Autodesk Inventor part; units mm, degrees
ref_plane "YZ Plane" through (0, 0, 0) normal (1, 0, 0) x (0, 1, 0)
ref_plane "XZ Plane" through (0, 0, 0) normal (0, 1, 0) x (-1, 0, 0)
ref_plane "XY Plane" through (0, 0, 0) normal (0, 0, 1) x (1, 0, 0)
sketch "Sketch1" plane through (0, 0, 0) normal (1, 0, 0) x (0, 1, 0)
  circle A0 centre (0, 0) radius 44
  dimension "d0" = 88
extrude "Extrusion1" add sketch "Sketch1" along normal blind 3.5
sketch "Sketch2" plane through (3.5, 0, 0) normal (1, 0, 0) x (0, 0, -1)
  circle A0 centre (0, 0) radius 45
  dimension "d3" = 90
extrude "Extrusion2" add sketch "Sketch2" along normal blind 1
sketch "Sketch3" plane through (0, 0, 0) normal (-1, 0, 0) x (0, 0, 1)
  circle A0 centre (0, 0) radius 45
  dimension "d6" = 90
extrude "Extrusion3" add sketch "Sketch3" along normal blind 1
sketch "Sketch4" plane through (4.5, 0, 0) normal (1, 0, 0) x (0, 0, -1)
  circle A0 centre (0, 0) radius 41.5
  dimension "d9" = 83
extrude "Extrusion4" cut sketch "Sketch4" against normal blind 6
sketch "Sketch5" plane through (4.5, 0, 0) normal (1, 0, 0) x (0, 0, -1)
  circle A0 centre (0, 0) radius 3.5
  dimension "d12" = 7
extrude "Extrusion5" add sketch "Sketch5" against normal blind 10
sketch "Sketch6" plane through (4.5, 0, 0) normal (1, 0, 0) x (0, 0, -1)
  circle A0 centre (0, 0) radius 45
extrude "Extrusion6" cut sketch "Sketch6" against normal blind 2
sketch "Sketch7" plane through (2.5, 0, 0) normal (1, 0, 0) x (0, 0, -1)
  circle A0 centre (0, 0) radius 3.5
  circle A1 centre (0, 0) radius 41.5
  circle A2 centre (0, 0) radius 45
extrude "Extrusion7" add sketch "Sketch7" along normal blind 1 contours A2
sketch "Sketch8" plane through (2.5, 0, 0) normal (1, 0, 0) x (0, 0, -1)
  circle A0 centre (0, 0) radius 3.5
extrude "Extrusion8" add sketch "Sketch8" along normal blind 1
sketch "Sketch9" plane through (3.5, 0, 0) normal (1, 0, 0) x (0, 0, -1)
  circle A0 centre (0, 0) radius 1.625
  dimension "d21" = 3.25
extrude "Extrusion9" cut sketch "Sketch9" against normal blind 10
sketch "Sketch10" plane through (3.5, 0, 0) normal (1, 0, 0) x (0, 0, -1)
  line L0 (2, 2.1756) -> (-2, 2.1756)
  line L1 (-2, 2.1756) -> (-2, 42.8244)
  line L2 (-2, 42.8244) -> (2, 42.8244)
  line L3 (2, 42.8244) -> (2, 2.1756)
  line L4 (2, 2.1756) -> (-2, 42.8244) construction
  line L5 (-2, 2.1756) -> (2, 42.8244) construction
  point P0 (0, 0)
  point P1 (0, 22.5)
  dimension "d24" = 4
extrude "Extrusion10" add sketch "Sketch10" against normal blind 4.5
pattern_circular "Circular Pattern1" count 4 over 360 about axis through (4.5, 0, 0) along (-1, 0, 0) of "Extrusion10"
fillet "Fillet1" radius 2 5 edges at (-1, 0, 3.5) (-1, -3.5, 0) (-1, 3.5, 0) (-1, -1.0481, -3.3394) (-1, 1.0481, -3.3394)
sketch "Sketch11" plane through (-5.5, 0, 0) normal (-1, 0, 0) x (0, 0, 1)
  circle A0 centre (0, 0) radius 1.625
  circle A1 centre (0, 0) radius 3.5
extrude "Extrusion11" add sketch "Sketch11" along normal blind 2
sketch "Sketch12" plane through (-7.5, 0, 0) normal (-1, 0, 0) x (0, 0, 1)
  circle A0 centre (0, 0) radius 1.625
  circle A1 centre (0, 0) radius 2
  dimension "d33" = 4
extrude "Extrusion12" add sketch "Sketch12" along normal blind 3.3
sketch "Sketch13" plane through (-10.8, 0, 0) normal (-1, 0, 0) x (0, 0, 1)
  circle A0 centre (0, 0) radius 3.5
  line L0 (2.5211, -2.4277) -> (-2.5211, -2.4277)
  line L1 (-2.5211, -2.4277) -> (-2.5211, 2.4277)
  line L2 (-2.5211, 2.4277) -> (2.5211, 2.4277)
  line L3 (2.5211, 2.4277) -> (2.5211, -2.4277)
  line L4 (2.5211, -2.4277) -> (-2.5211, 2.4277) construction
  line L5 (-2.5211, -2.4277) -> (2.5211, 2.4277) construction
extrude "Extrusion13" cut sketch "Sketch13" against normal blind 3.3 contours L3 L0 L1 L2
properties part number "mtv_pushingWheel_2-25"
The model under review builds one solid part; all positions refer to its coordinate system, in mm. A direction names the side the tool comes from. Give positions to 0.01 mm unless a question says otherwise; leave off trailing zeros. Order: outer loops, then holes, each group sorted by start corner. A loop starts at its lowest first (then second) coordinate and runs counter-clockwise, first axis right, second up. Notation, with made-up numbers: (44, 40.5) -> (82, 40.5) arc R20 ccw to (82, 59.5) -> close; hole circle Ø11 at (78.5, -8). An arc over 180 degrees is marked (long way). Write item = value, one per line. Start each with the question number.
(1) For L1, parallel to Y at x = -6, z = 0 (3 decimals); L2, parallel to Z at x = 2, y = 33; L3, parallel to Z at x = 2.75, y = -38, list the stretches that pass through material, from the lowest coordinate up. Write a range as from..to.
(2) Take a section at A-A (z = 0). Write out the cut boundary in (x, y) (3 decimals), plus the area to 3 significant figures.
(3) Tool access review of faces 1 (the flat face through (3.5, 0, -3)), 2 (the flat face through (1, -22, 2)), 3 (the cylindrical face through (1.232, -9.538, 42.954)): name each direction out of +Z, -Z, +X, -X, +Y, -Y from which nothing blocks a thin tool from reaching the whole face with its end or side.
(4) For pin 1 Ø3 at (x, z) = (-2, 19.5) entering from -Y; pin 2 Ø3.5 at (x, z) = (1, -19) entering from -Y; pin 3 Ø5 at (x, y) = (-1, 18.5) entering from +Z; pin 4 Ø2.5 at (y, z) = (0, 0) entering from -X, all flat-tipped, find the tip position at first contact; note any pin that passes through.
(5) Take a section at C-C (z = -39). Write out the cut boundary in (x, y).
(6) Draft analysis for pull direction X (two halves, no side actions). For faces 4 (the flat face through (0, -9.8, 43.1)), 5 (the flat face through (-1, -6, 0)), 6 (the flat face through (1, -2, -22)), state which applies: +X half, -X half, draft (parallel to the pull), parting line (faces both ways), or undercut.
(7) Take a section at B-B (y = -20.5). Write out the cut boundary in (x, z), plus the area to 3 significant figures.
Returned:
q1.L1 = -3.5..-1.625, 1.625..3.5
q1.L2 = -29.1..-25.16, -2..2, 25.16..29.1
q1.L3 = -24.1..-16.68, -2..2, 16.68..24.1
q2.outline = (-7.5, -3.5) -> (-3, -3.5) arc R2 cw to (-1, -5.5) -> (-1, -45) -> (0, -45) -> (0, -44) -> (2.5, -44) -> (2.5, -45) -> (3.5, -45) -> (3.5, -1.625) -> (-7.5, -1.625) -> close; (-7.5, 1.625) -> (3.5, 1.625) -> (3.5, 45) -> (2.5, 45) -> (2.5, 44) -> (0, 44) -> (0, 45) -> (-1, 45) -> (-1, 5.5) arc R2 cw to (-3, 3.5) -> (-7.5, 3.5) -> close
q2.area = 411 mm²
q3.face_1 = +Z, -Z, +X, +Y, -Y
q3.face_2 = +X, -X
q3.face_3 = none
q4.pin_1 = -41.07
q4.pin_2 = -41.43
q4.pin_3 = 42.06
q4.pin_4 = through
q5.outline = (-1, -22.45) -> (0, -22.45) -> (0, -20.37) -> (2.5, -20.37) -> (2.5, -22.45) -> (3.5, -22.45) -> (3.5, -14.19) -> (-1, -14.19) -> close; (-1, -2) -> (3.5, -2) -> (3.5, 2) -> (-1, 2) -> close; (-1, 14.19) -> (3.5, 14.19) -> (3.5, 22.45) -> (2.5, 22.45) -> (2.5, 20.37) -> (0, 20.37) -> (0, 22.45) -> (-1, 22.45) -> close
q6.face_4 = undercut
q6.face_5 = -X half
q6.face_6 = draft
q7.outline = (-1, -40.06) -> (0, -40.06) -> (0, -38.93) -> (2.5, -38.93) -> (2.5, -40.06) -> (3.5, -40.06) -> (3.5, -36.08) -> (-1, -36.08) -> close; (-1, -2) -> (3.5, -2) -> (3.5, 2) -> (-1, 2) -> close; (-1, 36.08) -> (3.5, 36.08) -> (3.5, 40.06) -> (2.5, 40.06) -> (2.5, 38.93) -> (0, 38.93) -> (0, 40.06) -> (-1, 40.06) -> close
q7.area = 48.2 mm²
